```python
from build123d import *

# Parameters (mm, degrees)
SKETCH1_W           = 71
SKETCH1_H           = 71
SKETCH1_R           = 1.5
SKETCH1_R_2         = 4.75
BOSS_EXTRUDE1_DEPTH = 5
FILLET1_R           = 8


with BuildPart() as part:
    # Sketch1 → Boss-Extrude1 (new body)
    with BuildSketch(Plane(origin=(0, 0, 0), x_dir=(1, 0, 0), z_dir=(0, 1, 0))):
        with Locations((35.5, 35.5)):
            Rectangle(SKETCH1_W, SKETCH1_H)
        with Locations((6, 6)):
            Circle(SKETCH1_R, mode=Mode.SUBTRACT)
        with Locations((65, 6)):
            Circle(SKETCH1_R, mode=Mode.SUBTRACT)
        with Locations((65, 65)):
            Circle(SKETCH1_R, mode=Mode.SUBTRACT)
        with Locations((6, 65)):
            Circle(SKETCH1_R, mode=Mode.SUBTRACT)
        with Locations((35.5, 35.5)):
            Circle(SKETCH1_R_2, mode=Mode.SUBTRACT)
    extrude(amount=BOSS_EXTRUDE1_DEPTH)

    # Fillet1
    fillet1_edges = [part.edges().sort_by_distance(p)[0] for p in [
        (0, 2.5, -71),
        (71, 2.5, -71),
        (71, 2.5, 0),
        (0, 2.5, 0),
    ]]
    fillet(fillet1_edges, radius=FILLET1_R)


solid = part.part
```
Geometry: final body of the model. Coordinates: model frame, mm. Round coordinates to 2 decimals unless told otherwise and drop trailing zeros. Order: outer loops, then holes, each group sorted by start corner. A loop starts at its lowest first (then second) coordinate and runs counter-clockwise, first axis right, second up. Notation, with made-up numbers: (46, -6.5) -> (79, -6.5) arc R36 cw to (79, 30.5) -> close; hole circle Ø10 at (35.25, -11.5). An arc over 180 degrees is marked (long way). Use one line per item in the form item = value. Start each with the question number.
1. Line query: probe 1 along X at (y, z) = (2.6, -35.5); probe 2 along X at (y, z) = (3.6, -65); probe 3 along Z at (x, y) = (6, 1.85). Output: solid intervals per line, ascending.
2. Draft query along Z for faces 1 (the face through (35, 2, -71)), 2 (the face through (27, 0, -36)), 3 (the face through (4.8, 2.5, -5.1)). Return one class per face: pulls with the +Z half, pulls with the -Z half, needs draft (parallel to the pull), parting line crosses it, or undercut.
3. Cut plane D-D (x = 65). Return the cut outline in (y, z), then the cut area to 3 significant figures.
4. Cut plane A-A (x = 35.5). Return the cut outline in (y, z).
5. Cut plane C-C (z = -65). Return the cut outline in (x, y).
6. Cut plane B-B (y = 4.05). Return the cut outline in (x, z).
Solution:
q1.probe_1 = 0 to 30.75, 40.25 to 71
q1.probe_2 = 0.25 to 4.5, 7.5 to 63.5, 66.5 to 70.75
q1.probe_3 = -70.75 to -66.5, -63.5 to -7.5, -4.5 to -0.25
q2.face_1 = pulls with the -Z half
q2.face_2 = needs draft
q2.face_3 = undercut
q3.outline = (0, -70.75) -> (5, -70.75) -> (5, -66.5) -> (0, -66.5) -> close; (0, -63.5) -> (5, -63.5) -> (5, -7.5) -> (0, -7.5) -> close; (0, -4.5) -> (5, -4.5) -> (5, -0.25) -> (0, -0.25) -> close
q3.area = 322 mm^2
q4.outline = (0, -71) -> (5, -71) -> (5, -40.25) -> (0, -40.25) -> close; (0, -30.75) -> (5, -30.75) -> (5, 0) -> (0, 0) -> close
q5.outline = (0.25, 0) -> (4.5, 0) -> (4.5, 5) -> (0.25, 5) -> close; (7.5, 0) -> (63.5, 0) -> (63.5, 5) -> (7.5, 5) -> close; (66.5, 0) -> (70.75, 0) -> (70.75, 5) -> (66.5, 5) -> close
q6.outline = (0, -63) arc R8 ccw to (8, -71) -> (63, -71) arc R8 ccw to (71, -63) -> (71, -8) arc R8 ccw to (63, 0) -> (8, 0) arc R8 ccw to (0, -8) -> close; hole circle Ø3 at (6, -65); hole circle Ø3 at (6, -6); hole circle Ø9.5 at (35.5, -35.5); hole circle Ø3 at (65, -65); hole circle Ø3 at (65, -6)
